Source: CAD feature listing. Evaluate the final solid. Frame: model axes, mm. Face numbers are marked on the shaded views. Give positions to 0.01 mm unless a question says otherwise; leave off trailing zeros. Write each loop counter-clockwise with the first axis right and the second up, starting at its lowest first coordinate (ties: lowest second). Pieces come first, ordered by that corner, then holes. Notation, with made-up numbers: (59.25, -1) -> (84.25, -1) arc R10 ccw to (84.25, 17) -> close; hole circle Ø4 at (-16.5, 38). An arc over 180 degrees is marked (long way). Use one line per item in the form item = value. Start each with the question number.
(1) Material intervals for line 1 along Z through (x, y) = (-0.25, 0); line 2 along Y through (x, z) = (8.75, 7); line 3 along Z through (x, y) = (10, -3), sorted ascending. Write a range as from..to.
(2) Cut plane A-A, the plane z = 6. Output: boundary loops of the cut face in (x, y).
(3) First-contact query: P1, Ø8, axis at y = 0, z = 6, coming from the -X side; P2, Ø6, axis at x = 11, y = 5, coming from the +Z side; P3, Ø3, axis at x = 7.5, y = -11, coming from the +Z side. Flat tips, straight axial feed; report the tip coordinate or a pass-through.
(4) Draft query along Z for the marked faces 1, 2, 3 and 4. Return one class per face: pulls with the +Z half, pulls with the -Z half, needs draft (parallel to the pull), parting line crosses it, or undercut.
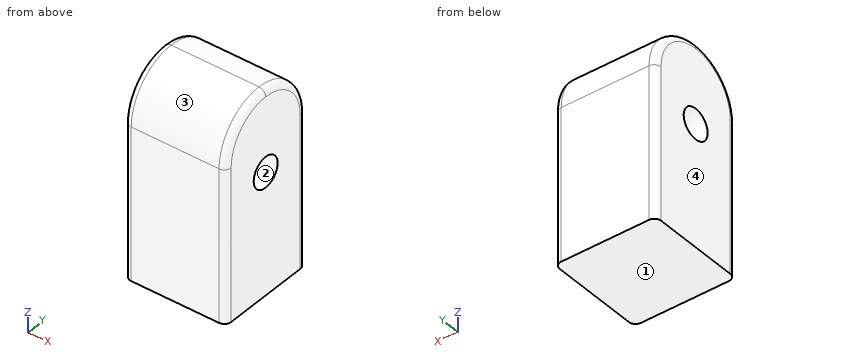
from build123d import *

# Parameters (mm, degrees)
F0_W     = 30
F0_H     = 60
F1_DEPTH = 15
F3_R     = 14.99999
F4_R     = 2
F5_D     = 9


# Not quite as in the source:
# - a fillet or chamfer is up to 0.001 mm smaller than in the source, because OpenCascade refuses the exact size


with BuildPart() as f1:
    # F0 (on Right) → F1 (new body, symmetric)
    with BuildSketch(Plane.YZ):
        Rectangle(F0_W, F0_H)
    extrude(amount=F1_DEPTH, both=True)

    # F3 (radius 15 in the source; OpenCascade refuses exactly that, so slightly less here)
    f3_edges = [f1.edges().sort_by_distance(p)[0] for p in [
        (0, -15, 30),
        (0, 15, 30),
    ]]
    fillet(f3_edges, radius=F3_R)

    # F4
    f4_edges = [f1.edges().sort_by_distance(p)[0] for p in [
        (15, -15, -7.499995),
        (-15, 15, -7.499995),
        (-15, -10.606605, 25.606605),
    ]]
    fillet(f4_edges, radius=F4_R)

    # F5 (through all)
    with Locations(Plane.YZ.offset(15)):
        with Locations((0, 6)):
            Hole(F5_D / 2)


solid = f1.part
Geometry says:
q1.line_1 = -30..1.5, 10.5..30
q1.line_2 = -15..-4.39, 4.39..15
q1.line_3 = -30..2.65, 9.35..29.7
q2.outline = (-15, -13) arc R2 ccw to (-13, -15) -> (13, -15) arc R2 ccw to (15, -13) -> (15, -4.5) -> (-15, -4.5) -> close; (-15, 4.5) -> (15, 4.5) -> (15, 13) arc R2 ccw to (13, 15) -> (-13, 15) arc R2 ccw to (-15, 13) -> close
q3.P1 = through
q3.P2 = 29.87
q3.P3 = 26.61
q4.face_1 = pulls with the -Z half
q4.face_2 = undercut
q4.face_3 = pulls with the +Z half
q4.face_4 = needs draft
